Autodesk Inventor part; units mm, degrees
ref_plane "YZ Plane" through (0, 0, 0) normal (1, 0, 0) x (0, 1, 0)
ref_plane "XZ Plane" through (0, 0, 0) normal (0, 1, 0) x (-1, 0, 0)
ref_plane "XY Plane" through (0, 0, 0) normal (0, 0, 1) x (1, 0, 0)
sketch "Sketch1" plane through (0, 0, 0) normal (0, 0, 1) x (1, 0, 0)
  point P0 (0, 0)
sketch "Sketch2" plane through (0, 0, 0) normal (0, 0, 1) x (1, 0, 0)
  line L0 (0, 0) -> (150.622, 0)
  line L1 (150.622, 0) -> (150.622, 304.8)
  line L2 (150.622, 304.8) -> (0, 304.8)
  line L3 (0, 304.8) -> (0, 0)
  circle A0 centre (25.4, 279.4) radius 3.9687
  circle A1 centre (125.222, 279.4) radius 3.9687
  circle A2 centre (25.4, 25.4) radius 3.9688
  circle A3 centre (125.222, 25.4) radius 3.9688
  dimension "d0" = 150.622
  dimension "d1" = 304.8
  dimension "d2" = 7.9375
  dimension "d3" = 25.4
  dimension "d4" = 25.4
  dimension "d5" = 7.9375
  dimension "d6" = 25.4
  dimension "d7" = 25.4
  dimension "d8" = 7.9375
  dimension "d9" = 25.4
  dimension "d10" = 25.4
  dimension "d11" = 7.9375
  dimension "d12" = 25.4
  dimension "d13" = 25.4
extrude "Extrusion1" add sketch "Sketch2" along normal blind 12.7
sketch "Sketch3" plane through (0, 0, 12.7) normal (0, 0, 1) x (1, 0, 0)
  line L0 (150.622, 304.8) -> (0, 304.8)
  line L1 (0, 0) -> (150.622, 0)
  line L2 (0, 304.8) -> (0, 0)
  line L3 (150.622, 0) -> (150.622, 304.8)
  circle A0 centre (57.811, 76.2) radius 1.905
  circle A1 centre (75.311, 93.7) radius 1.905
  circle A2 centre (75.311, 58.7) radius 1.905
  circle A3 centre (92.811, 76.2) radius 1.905
  point P0 (75.311, 76.2)
  dimension "d16" = 228.6
  dimension "d17" = 76.2
  dimension "d18" = 75.311
  dimension "d19" = 75.311
  dimension "d31" = 3.81
  dimension "d32" = 3.81
  dimension "d33" = 3.81
  dimension "d34" = 3.81
  dimension "d45" = 34.9999
  dimension "d46" = 17.5
  dimension "d47" = 17.5
  dimension "d48" = 17.5
hole "Hole1" at (75.311, 76.2, 12.7) direction (0, 0, -1) diameter 13.97 end through all
extrude "Extrusion2" cut sketch "Sketch3" against normal blind 25.4 contours A0 | A1 | A2 | A3
Model file for the job. Use its own axes, mm. Give positions to 0.01 mm unless a question says otherwise; leave off trailing zeros. Loops run counter-clockwise (first coordinate to the right, second up) from the corner with the lowest first, then second, coordinate; pieces in that order, holes last.
1) Flat gauge pin, fed straight in: pin 1 Ø6.5 at (x, y) = (25.4, 25.4) entering from -Z. Where does the tip first touch, or does it go through?
2) Pull direction Y, two halves, no side cores. Call faces 1 (the flat face through (74, 155, 0)), 2 (the cylindrical face through (77.99, 69.75, 6.26)), 3 (the flat face through (76, 304.8, 6)): +Y half, -Y half, draft (parallel to the pull), parting line (faces both ways), or undercut.
3) Wall check: line 1 (Y direction, x = 25.4, z = 9.25); line 2 (X direction, y = 279.4, z = 4.75); line 3 (X direction, y = 93.7, z = 4.25). Give the ranges that are in metal, low to high.
4) Saw through at A-A (y = 25.4). Write the cut outline in (x, z).
Answer block:
1. pin 1: passes through
2. face 1: draft
2. face 2: undercut
2. face 3: +Y half
3. line 1: y = 0 to 21.43, 29.37 to 275.43, 283.37 to 304.8
3. line 2: x = 0 to 21.43, 29.37 to 121.25, 129.19 to 150.62
3. line 3: x = 0 to 73.41, 77.22 to 150.62
4. outline: (0, 0) - (21.43, 0) - (21.43, 12.7) - (0, 12.7) - close; (29.37, 0) - (121.25, 0) - (121.25, 12.7) - (29.37, 12.7) - close; (129.19, 0) - (150.62, 0) - (150.62, 12.7) - (129.19, 12.7) - close
